For this review, take the finished solid that the model builds, in its own axes (mm). A direction names the side the tool comes from. Coordinates: 2 decimals unless noted, no trailing zeros. Loops run counter-clockwise (first coordinate to the right, second up) from the corner with the lowest first, then second, coordinate; pieces in that order, holes last. Notation, with made-up numbers: (8.5, 31.5) -> (27.5, 31.5) arc R16 cw to (27.5, 42.5) -> close; hole circle Ø7 at (81.25, 13). An arc over 180 degrees is marked (long way). Answer in a Markdown table with one row per item.
from build123d import *

# Parameters (mm, degrees)
SKETCH1_W           = 63.5
SKETCH1_H           = 88.9
BOSS_EXTRUDE1_DEPTH = 6.35
SKETCH2_R           = 1.5
BOSS_EXTRUDE2_DEPTH = 12


with BuildPart() as part:
    # Sketch1 → Boss-Extrude1 (new body)
    with BuildSketch(Plane(origin=(0, 0, 0), x_dir=(1, 0, 0), z_dir=(0, 1, 0))):
        Rectangle(SKETCH1_W, SKETCH1_H)
    extrude(amount=BOSS_EXTRUDE1_DEPTH)

    # Sketch2 → Boss-Extrude2 (add)
    with BuildSketch(Plane(origin=(0, 6.35, 0), x_dir=(1, 0, 0), z_dir=(0, 1, 0))):
        with Locations(Location((-27.5, 42.547666838, 0), (0, 0, 270))):
            Circle(SKETCH2_R)
        with Locations(Location((27.5, 42.547666838, 0), (0, 0, 270))):
            Circle(SKETCH2_R)
        with Locations(Location((27.5, -42.547666838, 0), (0, 0, 270))):
            Circle(SKETCH2_R)
        with Locations(Location((-27.5, -42.547666838, 0), (0, 0, 270))):
            Circle(SKETCH2_R)
    extrude(amount=BOSS_EXTRUDE2_DEPTH)


solid = part.part
Item 1: Take a section at D-D, the plane x = -22. State the section outline as (y, z) points.
Worked answers:
| item | result |
|---|---|
| outline | (0, -44.45) -> (6.35, -44.45) -> (6.35, 44.45) -> (0, 44.45) -> close |
Item 2: Take a section at A-A, the plane x = 27.5. State the section outline as (y, z) points.
Worked answers:
| item | result |
|---|---|
| outline | (0, -44.45) -> (6.35, -44.45) -> (6.35, -44.05) -> (18.35, -44.05) -> (18.35, -41.05) -> (6.35, -41.05) -> (6.35, 41.05) -> (18.35, 41.05) -> (18.35, 44.05) -> (6.35, 44.05) -> (6.35, 44.45) -> (0, 44.45) -> close |
Item 3: For L1, parallel to Y at x = -21, z = -13; L2, parallel to Z at x = 26.5, y = 14; L3, parallel to Z at x = -27, y = 9.25, list the stretches that pass through material, from the lowest coordinate up.
Worked answers:
| item | result |
|---|---|
| L1 | 0 to 6.35 |
| L2 | -43.67 to -41.43, 41.43 to 43.67 |
| L3 | -43.96 to -41.13, 41.13 to 43.96 |
Item 4: Take a section at C-C, the plane z = -22. State the section outline as (x, y) points, and give its area (3 significant figures).
Worked answers:
| item | result |
|---|---|
| outline | (-31.75, 0) -> (31.75, 0) -> (31.75, 6.35) -> (-31.75, 6.35) -> close |
| area | 403 mm² |
Item 5: The part is to be moulded in two halves that separate along X. For faces 1 (the flat face through (28, 18.35, 43)), 2 (the cylindrical face through (28.987, 12.266, -42.743)), 3 (the flat face through (31.75, 3, 1)), say which applies: +X half, -X half, draft (parallel to the pull), parting line (faces both ways), or undercut.
Worked answers:
| item | result |
|---|---|
| face 1 | draft |
| face 2 | undercut |
| face 3 | +X half |
Item 6: Take a section at B-B, the plane y = 12. State the section outline as (x, z) points, and give its area (3 significant figures).
Worked answers:
| item | result |
|---|---|
| outline | circle Ø3 at (-27.5, -42.55); circle Ø3 at (-27.5, 42.55); circle Ø3 at (27.5, -42.55); circle Ø3 at (27.5, 42.55) |
| area | 28.3 mm² |
Item 7: Insertion check: pin 1 (19 mm diameter, centred on x = -13, z = 19, fed in from +Y); pin 2 (2 mm diameter, centred on x = 16, z = -21.5, fed in from -Y). Each pin has a flat end and moves straight along its axis. Give the tip position at first contact, or say it passes through.
Worked answers:
| item | result |
|---|---|
| pin 1 | y = 6.35 |
| pin 2 | y = 0 |
Item 8: For faces 4 (the flat face through (-31.75, 3, 1)), 5 (the cylindrical face through (-27.05, 12.27, 43.98)), list the 3-axis set-ups (+Z, -Z, +X, -X, +Y, -Y) from which the entire face can be reached by the end or side of a thin tool; tool diameter is ignored.
Worked answers:
| item | result |
|---|---|
| face 4 | +Z, -Z, -X, +Y, -Y |
| face 5 | +Y |
